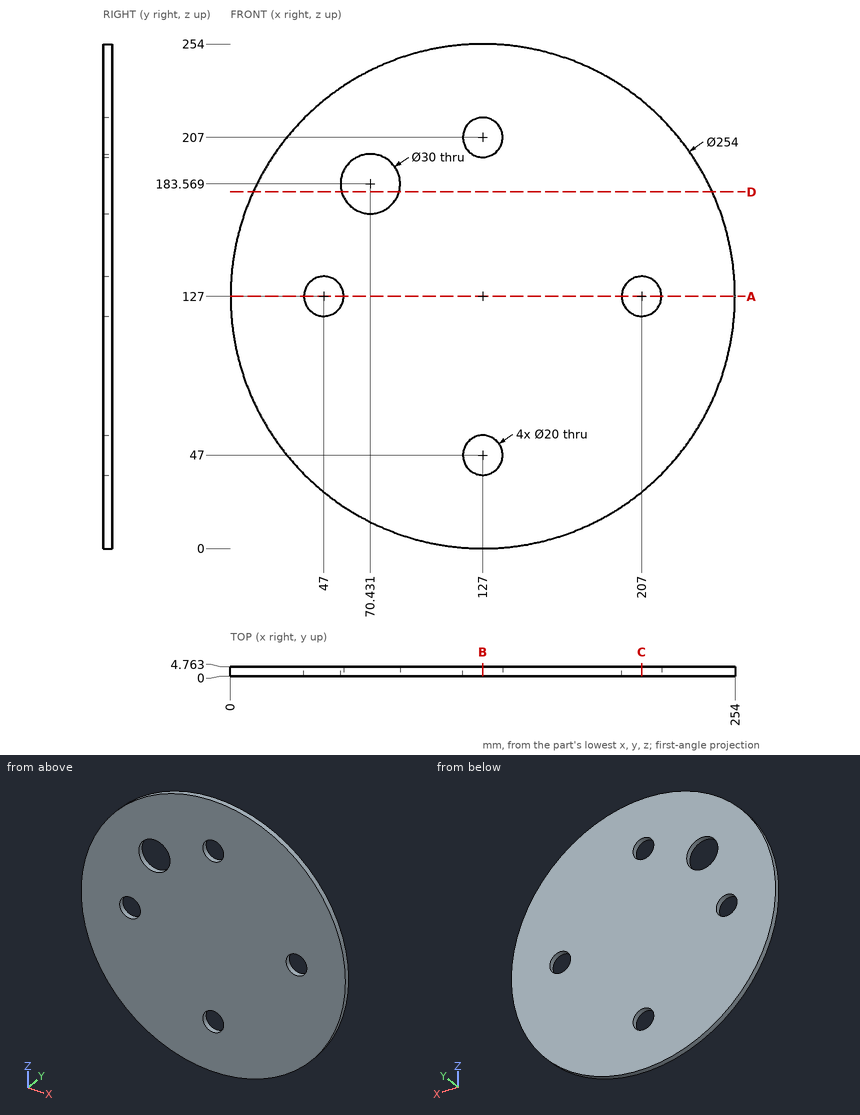
Input: dimensioned drawing with shaded views. Units: mm. Origin: part minimum x, y, z. Round coordinates to 2 decimals unless told otherwise and drop trailing zeros. Order: outer loops, then holes, each group sorted by start corner. A loop starts at its lowest first (then second) coordinate and runs counter-clockwise, first axis right, second up. Notation, with made-up numbers: (64.25, 62.25) - (116.25, 62.25) arc R29 cw to (116.25, 89.25) - close; hole circle Ø7 at (75, 4.5). An arc over 180 degrees is marked (long way). Answer as a JSON object with one key per item and string values. Group by question number.
(1) Cut plane C-C (x = 207). Return loops of the section in (y, z) (1 decimal).
(2) Cut plane B-B (x = 127). Return loops of the section in (y, z), then the cut area to 3 significant figures.
(3) Material intervals for probe 1 along Z at (x, y) = (127, 1.9); probe 2 along X at (y, z) = (1.2, 170.5) (1 decimal); probe 3 along Z at (x, y) = (207, 1.6) (1 decimal), sorted ascending. Write a range as from..to.
(4) Cut plane A-A (z = 127). Return loops of the section in (x, y), then the cut area to 3 significant figures.
(5) Cut plane D-D (z = 179.5). Return loops of the section in (x, y), then the cut area to 3 significant figures.
(6) Pin query (flat end, axial travel): P1, Ø2, axis at y = 2, z = 139.5, coming from the +X side; P2, Ø16, axis at x = 127, z = 47, coming from the +Y side. Return the tip coordinate at first contact, or that it passes through.
Here are the results:
{
 "1": {"outline": "(0, 28.4) - (4.8, 28.4) - (4.8, 117) - (0, 117) - close; (0, 137) - (4.8, 137) - (4.8, 225.6) - (0, 225.6) - close"},
 "2": {"outline": "(0, 0) - (4.76, 0) - (4.76, 37) - (0, 37) - close; (0, 57) - (4.76, 57) - (4.76, 197) - (0, 197) - close; (0, 217) - (4.76, 217) - (4.76, 254) - (0, 254) - close", "area": "1,020 mm^2"},
 "3": {"probe 1": "z = 0..37, 57..197, 217..254", "probe 2": "x = 7.7..63.1, 77.8..246.3", "probe 3": "z = 28.4..117, 137..225.6"},
 "4": {"outline": "(0, 0) - (37, 0) - (37, 4.76) - (0, 4.76) - close; (57, 0) - (197, 0) - (197, 4.76) - (57, 4.76) - close; (217, 0) - (254, 0) - (254, 4.76) - (217, 4.76) - close", "area": "1,020 mm^2"},
 "5": {"outline": "(11.36, 0) - (55.99, 0) - (55.99, 4.76) - (11.36, 4.76) - close; (84.87, 0) - (242.64, 0) - (242.64, 4.76) - (84.87, 4.76) - close", "area": "964 mm^2"},
 "6": {"P1": "stops at x = 253.48", "P2": "passes through"}
}
